from build123d import *

# Parameters (mm, degrees)
SKETCH1_W           = 167.64
SKETCH1_H           = 137.16
BOSS_EXTRUDE1_DEPTH = 12.7
SKETCH2_W           = 167.64
SKETCH2_H           = 91.44
CUT_EXTRUDE1_DEPTH  = 7.62
SKETCH3_W           = 5.08
SKETCH3_H           = 22.86
CUT_EXTRUDE2_DEPTH  = 2.286
SKETCH4_R           = 6.35
SKETCH4_R_2         = 4.826
BOSS_EXTRUDE2_DEPTH = 30.464799878
SKETCH5_W           = 167.64
SKETCH5_H           = 7.62
BOSS_EXTRUDE3_DEPTH = 30.464799878
FILLET1_R           = 19.05
FILLET2_R           = 10.16


with BuildPart() as part:
    # Sketch1 → Boss-Extrude1 (new body)
    with BuildSketch(Plane(origin=(0, 0, 0), x_dir=(1, 0, 0), z_dir=(0, 1, 0))):
        with Locations((83.82, 68.58)):
            Rectangle(SKETCH1_W, SKETCH1_H)
    extrude(amount=BOSS_EXTRUDE1_DEPTH)

    # Sketch2 → Cut-Extrude1 (cut)
    with BuildSketch(Plane(origin=(0, 12.7, 0), x_dir=(1, 0, 0), z_dir=(0, 1, 0))):
        with Locations((83.82, 68.58)):
            Rectangle(SKETCH2_W, SKETCH2_H)
    extrude(amount=-CUT_EXTRUDE1_DEPTH, mode=Mode.SUBTRACT)

    # Sketch3 → Cut-Extrude2 (cut)
    with BuildSketch(Plane(origin=(0, 12.7, 0), x_dir=(1, 0, 0), z_dir=(0, 1, 0))):
        with Locations((2.54, 125.73)):
            Rectangle(SKETCH3_W, SKETCH3_H)
        with Locations((165.1, 125.73)):
            Rectangle(SKETCH3_W, SKETCH3_H)
        with Locations((165.1, 11.43)):
            Rectangle(SKETCH3_W, SKETCH3_H)
        with Locations((2.54, 11.43)):
            Rectangle(SKETCH3_W, SKETCH3_H)
    extrude(amount=-CUT_EXTRUDE2_DEPTH, mode=Mode.SUBTRACT)

    # Sketch4 → Boss-Extrude2 (add)
    # profile 1 of 2: a face of its own
    with BuildSketch(Plane.XZ):
        with Locations(Location((81.788, -15.494, 0), (0, 0, 90))):
            Circle(SKETCH4_R)
        with Locations(Location((81.788, -15.494, 0), (0, 0, 90))):
            Circle(SKETCH4_R_2, mode=Mode.SUBTRACT)
    # profile 2 of 2: a face of its own
    with BuildSketch(Plane.XZ):
        with Locations(Location((81.788, -121.92, 0), (0, 0, 90))):
            Circle(SKETCH4_R)
        with Locations(Location((81.788, -121.92, 0), (0, 0, 90))):
            Circle(SKETCH4_R_2, mode=Mode.SUBTRACT)
    extrude(amount=BOSS_EXTRUDE2_DEPTH)

    # Sketch5 → Boss-Extrude3 (add)
    with BuildSketch(Plane.XZ):
        with Locations((83.82, -133.35)):
            Rectangle(SKETCH5_W, SKETCH5_H)
        with Locations((83.82, -3.81)):
            Rectangle(SKETCH5_W, SKETCH5_H)
    extrude(amount=BOSS_EXTRUDE3_DEPTH)

    # Fillet1
    fillet1_edges = [part.edges().sort_by_distance(p)[0] for p in [
        (83.82, 12.7, 0),
        (83.82, 12.7, -137.16),
    ]]
    fillet(fillet1_edges, radius=FILLET1_R)

    # Fillet2
    # the kernel refuses this fillet: 10.16 mm, written as the material it adds along each edge
    with BuildSketch(Plane(origin=(0, 0, -7.62), x_dir=(0, -1, 0), z_dir=(1, 0, 0))) as fillet2_piece_1_section:
        with BuildLine():
            CenterArc((FILLET2_R, FILLET2_R), FILLET2_R, 180, 90)
            Line((0, FILLET2_R), (0, 0))
            Line((0, 0), (FILLET2_R, 0))
        make_face()
    fillet2_piece_1 = extrude(amount=167.64, mode=Mode.PRIVATE)
    fillet2_piece_1 = fillet2_piece_1 - Plane(origin=(81.788, -7.490679749, -15.494), x_dir=(0, 0, 1), z_dir=(0, 1, 0)) * Cylinder(4.826, 376, mode=Mode.PRIVATE)
    add(fillet2_piece_1)
    with BuildSketch(Plane(origin=(0, 0, -129.54), x_dir=(0, 0, 1), z_dir=(1, 0, 0))) as fillet2_piece_2_section:
        with BuildLine():
            CenterArc((FILLET2_R, FILLET2_R), FILLET2_R, 180, 90)
            Line((0, FILLET2_R), (0, 0))
            Line((0, 0), (FILLET2_R, 0))
        make_face()
    fillet2_piece_2 = extrude(amount=167.64, mode=Mode.PRIVATE)
    fillet2_piece_2 = fillet2_piece_2 - Plane(origin=(81.788, -0.198114481, -121.92), x_dir=(0, 0, 1), z_dir=(0, 1, 0)) * Cylinder(4.826, 376, mode=Mode.PRIVATE)
    add(fillet2_piece_2)


solid = part.part
The listing builds one solid part. Answer for the finished solid, in the listing's coordinates (mm). A direction names the side the tool comes from. Round coordinates to 2 decimals unless told otherwise and drop trailing zeros. Write each loop counter-clockwise with the first axis right and the second up, starting at its lowest first coordinate (ties: lowest second). Pieces come first, ordered by that corner, then holes. Notation, with made-up numbers: M -22.5,18.25 L -3.5,18.25 A26 ccw -3.5,32.25 Z; hole C 83.25,67 d8. An arc over 180 degrees is marked long. Write each question's results on one line, items separated by ' | '. Start each with the question number.
Item 1: For faces 1 (the face through (83, -20, -129.54)), 2 (the face through (165, 10.414, -17)), 3 (the face through (79.881, -15.019, -115.863)), 4 (the face through (83, 9, -114.3)), determine the directions among +Z, -Z, +X, -X, +Y, -Y from which every point of the face is accessible in a straight line to the end or side of a thin tool.
Item 2: Straight lines are drawn through the part: L1, parallel to X at y = -1, z = -121.92; L2, parallel to Z at x = 104.5, y = -17.5; L3, parallel to Y at x = 123, z = -104.5. For each, find the intervals that lie inside material, in ascending order. Write a range as [from, to].
Item 3: Flat-ended cylindrical pins translate along their axes: pin 1 Ø0.7 at (y, z) = (12, -122.5) entering from -X; pin 2 Ø6 at (x, z) = (144, -102.5) entering from +Y; pin 3 Ø4 at (x, y) = (71, 10.5) entering from +Z. Find the tip coordinate at first contact, or state that the pin passes through.
Item 4: For a pull along Z with two mould halves and no side action, classify faces 5 (the face through (83, -20, -7.62)), 6 (the face through (81.509, -15.019, -21.838)), 7 (the face through (84.99, 7.27, -5.73)), 8 (the face through (165, 10.414, -121)) as pulls with the +Z half, pulls with the -Z half, needs draft (parallel to the pull), parting line crosses it, or undercut.
Item 5: A cutting plane is placed at D-D on z = -121.92. Write down the section's boundary in (x, y), and give its area (3 significant figures).
Item 6: A cutting plane is placed at B-B on x = 138.5. Write down the section's boundary in (y, z), and give its area (3 significant figures).
Item 7: A cutting plane is placed at A-A on y = -17. Write down the section's boundary in (x, z), and give its area (3 significant figures).
Item 8: A cutting plane is placed at C-C on y = 7. Write down the section's boundary in (x, z), and give its area (3 significant figures).
Check sheet entries:
1) face 1: +X, -X, -Y | face 2: +Z, -Z, +X, +Y | face 3: -Y | face 4: +X, -X, +Y
2) L1: [75.44, 76.96], [86.61, 88.14] | L2: [-137.16, -129.54], [-7.62, 0] | L3: [0, 5.08]
3) pin 1: x = 5.08 | pin 2: y = 5.08 | pin 3: z = -7.12
4) face 5: undercut | face 6: undercut | face 7: pulls with the +Z half | face 8: needs draft
5) outline: M 0,-0.32 L 75.44,-0.32 L 75.44,-30.46 L 76.96,-30.46 L 76.96,0 L 86.61,0 L 86.61,-30.46 L 88.14,-30.46 L 88.14,-0.32 L 167.64,-0.32 L 167.64,10.41 L 162.56,10.41 L 162.56,12.32 L 5.08,12.32 L 5.08,10.41 L 0,10.41 Z | area: 2,190 mm²
6) outline: M -30.46,-137.16 L -6.35,-137.16 A19.05 ccw 12.7,-118.11 L 12.7,-114.3 L 5.08,-114.3 L 5.08,-22.86 L 12.7,-22.86 L 12.7,-19.05 A19.05 ccw -6.35,0 L -30.46,0 L -30.46,-7.62 L -10.16,-7.62 A10.16 cw 0,-17.78 L 0,-119.38 A10.16 cw -10.16,-129.54 L -30.46,-129.54 Z | area: 1,400 mm²
7) outline: M 0,-137.16 L 167.64,-137.16 L 167.64,-129.54 L 0,-129.54 Z; M 0,-7.62 L 167.64,-7.62 L 167.64,0 L 0,0 Z; C 81.79,-121.92 d12.7; C 81.79,-15.49 d12.7; hole C 81.79,-121.92 d9.65; hole C 81.79,-15.49 d9.65 | area: 2,660 mm²
8) outline: M 0,-131.7 L 167.64,-131.7 L 167.64,-114.3 L 0,-114.3 Z; M 0,-22.86 L 167.64,-22.86 L 167.64,-5.46 L 0,-5.46 Z | area: 5,830 mm²
